Input: part model. Units: mm. Frame: model coordinates. Face numbers are marked on the shaded views. A direction names the side the tool comes from. Coordinates: 2 decimals unless noted, no trailing zeros. Order: outer loops, then holes, each group sorted by start corner. A loop starts at its lowest first (then second) coordinate and runs counter-clockwise, first axis right, second up. Notation, with made-up numbers: (11, 14.25) -> (18, 14.25) arc R16 ccw to (18, 28.25) -> close; hole circle Ø4 at (76.25, -27). An arc over 180 degrees is marked (long way). Use one line per item in the form item = value. Start each with the question number.
1) Section query B-B on y = 33.5. Output: boundary loops of the cut face in (x, z).
2) Ray query, line 1 along Z through (x, y) = (-2, -22); line 2 along Y through (x, z) = (12, 13); line 3 along Y through (x, z) = (0, 16). Return the intervals inside material, ascending.
3) Access query for the marked faces 1 and 2. Directions: +Z, -Z, +X, -X, +Y, -Y. A direction counts if a zero-diameter tool reaches every point of the face in a straight line with its end or side. Return the directions, or none.
4) Section query C-C on z = 22.5. Output: boundary loops of the cut face in (x, y).
5) Pin query (flat end, axial travel): pin 1 (10 mm diameter, centred on x = 13.5, z = 25.5, fed in from -Y); pin 2 (1 mm diameter, centred on x = -19, z = 22, fed in from +Y); pin 3 (5.5 mm diameter, centred on y = -22.5, z = 15, fed in from +X). Return the tip coordinate at first contact, or that it passes through.
from build123d import *

# Parameters (mm, degrees)
EXTRUDE_1_DEPTH     = 30
SKETCH_2_R          = 3
CUT_EXTRUDE_1_DEPTH = 52
FILLET_1_R          = 15
FILLET_2_R          = 15
FILLET_3_R          = 15
FILLET_4_R          = 15
SKETCH_4_R          = 3
SKETCH_4_R_2        = 0.5
EXTRUDE_2_DEPTH     = 50


with BuildPart() as part:
    # 草图1 → 凸台-拉伸1 (new body)
    with BuildSketch(Plane.XY):
        Polygon((25, 0), (25, 42.5), (-25, 42.5), (-25, -32.5), (25, -32.5), align=None)
    extrude(amount=EXTRUDE_1_DEPTH)

    # 草图2 → 切除-拉伸1 (cut)
    with BuildSketch(Plane(origin=(25, 0, 0), x_dir=(0, 0, -1), z_dir=(1, 0, 0))):
        with Locations((-15, -22.5)):
            Circle(SKETCH_2_R)
    extrude(amount=-CUT_EXTRUDE_1_DEPTH, mode=Mode.SUBTRACT)

    # 圆角1
    fillet_1_edges = [part.edges().sort_by_distance(p)[0] for p in [
        (0, -32.5, 0),
    ]]
    fillet(fillet_1_edges, radius=FILLET_1_R)

    # 圆角2
    fillet_2_edges = [part.edges().sort_by_distance(p)[0] for p in [
        (0, -32.5, 30),
    ]]
    fillet(fillet_2_edges, radius=FILLET_2_R - 0.0001)  # a hair under: the kernel refuses the full size

    # 圆角3
    fillet_3_edges = [part.edges().sort_by_distance(p)[0] for p in [
        (0, 42.5, 30),
    ]]
    fillet(fillet_3_edges, radius=FILLET_3_R)

    # 圆角4
    fillet_4_edges = [part.edges().sort_by_distance(p)[0] for p in [
        (0, 42.5, 0),
    ]]
    fillet(fillet_4_edges, radius=FILLET_4_R - 0.0001)  # a hair under: the kernel refuses the full size

    # 草图4 → 凸台-拉伸2 (add)
    with BuildSketch(Plane(origin=(0, 0, 0), x_dir=(1, 0, 0), z_dir=(0, 1, 0))):
        with Locations((0, -15)):
            Circle(SKETCH_4_R)
        with Locations((15, -15)):
            Circle(SKETCH_4_R_2)
        with Locations((-15, -15)):
            Circle(SKETCH_4_R_2)
    extrude(amount=EXTRUDE_2_DEPTH)


solid = part.part
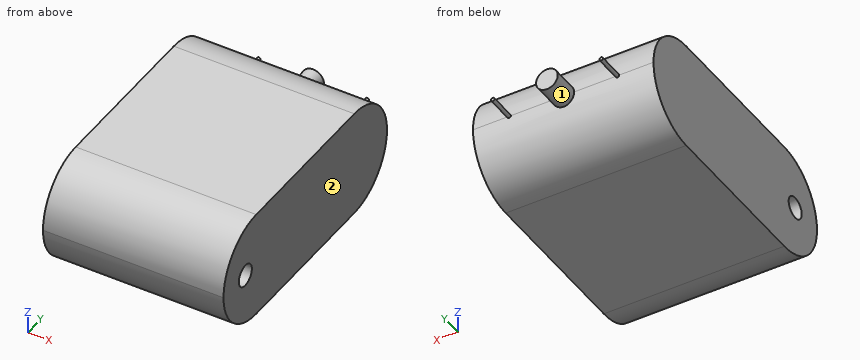
Answers below:
q1.outline = (-25, 1.25) -> (25, 1.25) -> (25, 28.75) -> (-25, 28.75) -> close
q2.line_1 = 0.69 to 12.04, 17.96 to 29.31
q2.line_2 = -32.37 to -24.74, -20.26 to 42.37
q2.line_3 = -32.47 to -25.33, -19.67 to 50
q3.face_1 = +Y
q3.face_2 = +Z, -Z, +X, +Y, -Y
q4.outline = (-25, -30.49) -> (25, -30.49) -> (25, 40.49) -> (-25, 40.49) -> close
q5.pin_1 = -31.46
q5.pin_2 = 41.02
q5.pin_3 = through
